```python
from build123d import *

# Parameters (mm, degrees)
EXTRUDE_1_DEPTH          = 70
CUT_EXTRUDE_1_DEPTH      = 100.498743711
SKETCH_4_W               = 45.819685342
SKETCH_4_H               = 5
CUT_EXTRUDE_2_DEPTH      = 96.72878355
SKETCH_5_W               = 32
SKETCH_5_H               = 10
SKETCH_5_H_2             = 40
CUT_EXTRUDE_3_DEPTH      = 94.214805691
CUT_EXTRUDE_4_DEPTH      = 1
SKETCH_7_R               = 3.75
CUT_EXTRUDE_5_DEPTH      = 10
CUT_EXTRUDE_6_REACH      = 97.729
SKETCH_8_R               = 2.5
CUT_EXTRUDE_7_DEPTH      = 92.782351245
CUT_EXTRUDE_7_DEPTH_BACK = 92.782351245
CUT_EXTRUDE_8_DEPTH      = 96
CHAMFER_1_SIZE           = 1


with BuildPart() as part:
    # 草图1 → 拉伸1 (new body)
    with BuildSketch(Plane.XY):
        Polygon((0, 0), (50, 0), (0, 50), align=None)
    extrude(amount=EXTRUDE_1_DEPTH)

    # 草图3 → 切除-拉伸1 (cut, through all)
    with BuildSketch(Plane.XY.offset(70)):
        Polygon((50, 0), (42, 0), (42, 8), align=None)
    extrude(amount=-CUT_EXTRUDE_1_DEPTH, mode=Mode.SUBTRACT)

    # 草图4 → 切除-拉伸2 (cut, through all)
    with BuildSketch(Plane.XY.offset(70)):
        with Locations((32.909842671, 2.5)):
            Rectangle(SKETCH_4_W, SKETCH_4_H)
    extrude(amount=-CUT_EXTRUDE_2_DEPTH, mode=Mode.SUBTRACT)

    # 草图5 → 切除-拉伸3 (cut, through all)
    with BuildSketch(Plane.XZ.offset(-5)):
        with Locations((26, 55)):
            Rectangle(SKETCH_5_W, SKETCH_5_H)
        with Locations((26, 20)):
            Rectangle(SKETCH_5_W, SKETCH_5_H_2)
    extrude(amount=-CUT_EXTRUDE_3_DEPTH, mode=Mode.SUBTRACT)

    # 草图6 → 切除-拉伸4 (cut)
    with BuildSketch(Plane.XY.offset(70)):
        Polygon((0, 50), (0, 30), (20, 30), align=None)
    extrude(amount=-CUT_EXTRUDE_4_DEPTH, mode=Mode.SUBTRACT)

    # 草图7 → 切除-拉伸5 (cut)
    with BuildSketch(Plane.XZ.offset(-5)):
        with Locations(Location((16, 65, 0), (0, 0, 270))):
            Circle(SKETCH_7_R)
    extrude(amount=-CUT_EXTRUDE_5_DEPTH, mode=Mode.SUBTRACT)

    # 切除-拉伸6: up to this face of the body (flat: up to its plane)
    cut_extrude_6_end = Plane(part.part.faces().sort_by_distance((21.50877193, 16.745614035, 40))[0])
    # 草图8 → 切除-拉伸6 (cut, up to the picked face)
    with BuildSketch(Plane.XY.offset(70), mode=Mode.PRIVATE) as cut_extrude_6_sk1:
        with Locations((5, 36)):
            Circle(SKETCH_8_R)
    cut_extrude_6_tool1 = split(extrude(cut_extrude_6_sk1.sketch, amount=-CUT_EXTRUDE_6_REACH, mode=Mode.PRIVATE), bisect_by=cut_extrude_6_end, keep=Keep.BOTH, mode=Mode.PRIVATE)
    # 草图8 → 切除-拉伸6 (cut, up to the picked face)
    with BuildSketch(Plane.XY.offset(70), mode=Mode.PRIVATE) as cut_extrude_6_sk2:
        with Locations((5, 10)):
            Circle(SKETCH_8_R)
    cut_extrude_6_tool2 = split(extrude(cut_extrude_6_sk2.sketch, amount=-CUT_EXTRUDE_6_REACH, mode=Mode.PRIVATE), bisect_by=cut_extrude_6_end, keep=Keep.BOTH, mode=Mode.PRIVATE)
    # 草图8 → 切除-拉伸6 (cut, up to the picked face)
    with BuildSketch(Plane.XY.offset(70), mode=Mode.PRIVATE) as cut_extrude_6_sk3:
        with Locations((31, 10)):
            Circle(SKETCH_8_R)
    cut_extrude_6_tool3 = split(extrude(cut_extrude_6_sk3.sketch, amount=-CUT_EXTRUDE_6_REACH, mode=Mode.PRIVATE), bisect_by=cut_extrude_6_end, keep=Keep.BOTH, mode=Mode.PRIVATE)
    # 草图8 → 切除-拉伸6 (cut, up to the picked face)
    with BuildSketch(Plane.XY.offset(70), mode=Mode.PRIVATE) as cut_extrude_6_sk4:
        with Locations((18, 23)):
            Circle(SKETCH_8_R)
    cut_extrude_6_tool4 = split(extrude(cut_extrude_6_sk4.sketch, amount=-CUT_EXTRUDE_6_REACH, mode=Mode.PRIVATE), bisect_by=cut_extrude_6_end, keep=Keep.BOTH, mode=Mode.PRIVATE)
    add(cut_extrude_6_tool1.solids().sort_by(Axis((5, 36, 70), (0, 0, -1)))[0], mode=Mode.SUBTRACT)
    add(cut_extrude_6_tool2.solids().sort_by(Axis((5, 10, 70), (0, 0, -1)))[0], mode=Mode.SUBTRACT)
    add(cut_extrude_6_tool3.solids().sort_by(Axis((31, 10, 70), (0, 0, -1)))[0], mode=Mode.SUBTRACT)
    add(cut_extrude_6_tool4.solids().sort_by(Axis((18, 23, 70), (0, 0, -1)))[0], mode=Mode.SUBTRACT)

    # 草图9 → 切除-拉伸7 (cut, two sides: drawn at the far end of the back side and taken through both)
    with BuildSketch(Plane(origin=(10, 0, 0), x_dir=(0, 0, -1), z_dir=(1, 0, 0)).offset(-CUT_EXTRUDE_7_DEPTH_BACK)):
        Polygon((182.046505341, 50), (0, 50), (-40, 50), (0, 5), (120.945115134, -131.063254526), (465.924736836, -247.479666759), (527.026127043, -66.416412233), align=None)
    extrude(amount=CUT_EXTRUDE_7_DEPTH + CUT_EXTRUDE_7_DEPTH_BACK, mode=Mode.SUBTRACT)

    # 草图10 → 切除-拉伸8 (cut, through all)
    with BuildSketch(Plane.XY.offset(69)):
        Polygon((0, 50), (0, 47), (3, 47), align=None)
    extrude(amount=-CUT_EXTRUDE_8_DEPTH, mode=Mode.SUBTRACT)

    # 倒角1
    chamfer_1_edges = [part.edges().sort_by_distance(p)[0] for p in [
        (26, 5, 60),
        (26, 5, 50),
        (26, 5, 40),
    ]]
    chamfer(chamfer_1_edges, length=CHAMFER_1_SIZE)


solid = part.part
```
Here's how the part is built. I have some questions about the finished solid (model axes, mm). A direction names the side the tool comes from. Round coordinates to 2 decimals unless told otherwise and drop trailing zeros. Loops run counter-clockwise (first coordinate to the right, second up) from the corner with the lowest first, then second, coordinate; pieces in that order, holes last. Notation, with made-up numbers: (31, 79.25) -> (44, 79.25) arc R24 ccw to (44, 97.25) -> close; hole circle Ø9 at (-7.75, -36). An arc over 180 degrees is marked (long way). Answer as CSV lines item,"result". Start each with the question number.
1. Imagine slicing it at C-C on y = 23. Write out the boundary of the cut face in (x, z), plus the area to 3 significant figures.
2. If we mould it in two halves opening along Y, with no side actions, what happens to faces 4 (the face through (22, 19, 40)), 5 (the face through (4.46, 33.56, 54.7)), 6 (the face through (18, 32, 46)), 7 (the face through (5, 10, 40))? For each: pulls with the +Y half, pulls with the -Y half, needs draft (parallel to the pull), parting line crosses it, or undercut.
3. For faces 1 (the face through (8, 37, 69)), 2 (the face through (5, 36, 40)), 3 (the face through (16, 15, 65)), which set-ups out of +Z, -Z, +X, -X, +Y, -Y let a thin tool reach every point of the face, with its end or its side?
4. I need wall thicknesses on probe 1 along Z at (x, y) = (18.5, 26.5); probe 2 along X at (y, z) = (4, 33); probe 3 along Y at (x, z) = (18, 47). Which ranges of each line are inside material? Lowest first, please. Write a range as from..to.
5. I'm going to push flat-ended pins straight in: P1, Ø20, axis at y = 26.5, z = 44.5, coming from the +X side; P2, Ø4.5, axis at x = 18, y = 23, coming from the +Z side; P3, Ø6, axis at x = 16, z = 65, coming from the -Y side; P4, Ø6, axis at x = 6.5, z = 41, coming from the -Y side. Where does each tip first touch, or does it pass through?
6. Imagine slicing it at B-B on x = 22.5. Write out the boundary of the cut face in (y, z), plus the area to 4 significant figures.
7. Imagine slicing it at A-A on x = 31. Write out the boundary of the cut face in (y, z), plus the area to 4 significant figures.
8. Imagine slicing it at D-D on y = 10. Write out the boundary of the cut face in (x, z), plus the area to 3 significant figures.
Solution:
1,outline,"(0, 16) -> (10, 16) -> (10, 40) -> (15.5, 40) -> (15.5, 50) -> (10, 50) -> (10, 60) -> (15.5, 60) -> (15.5, 70) -> (0, 70) -> close; (20.5, 40) -> (27, 40) -> (27, 50) -> (20.5, 50) -> close; (20.5, 60) -> (27, 60) -> (27, 70) -> (20.5, 70) -> close"
1,area,"780 mm²"
2,face 4,"needs draft"
2,face 5,"undercut"
2,face 6,"pulls with the +Y half"
2,face 7,"undercut"
3,face 1,"+Z, +X, -X, +Y"
3,face 2,"+Z"
3,face 3,"-Y"
4,probe 1,"40..50, 60..70"
4,probe 2,"0..10"
4,probe 3,"5..20.5, 25.5..32"
5,P1,"x = 33.5"
5,P2,"through"
5,P3,"y = 15"
5,P4,"y = 0"
6,outline,"(5, 41) -> (6, 40) -> (27.5, 40) -> (27.5, 50) -> (6, 50) -> (5, 49) -> close; (5, 61) -> (6, 60) -> (27.5, 60) -> (27.5, 70) -> (5, 70) -> close"
6,area,"448.5 mm²"
7,outline,"(5, 41) -> (6, 40) -> (7.5, 40) -> (7.5, 50) -> (6, 50) -> (5, 49) -> close; (5, 61) -> (6, 60) -> (7.5, 60) -> (7.5, 70) -> (5, 70) -> close; (12.5, 40) -> (19, 40) -> (19, 50) -> (12.5, 50) -> close; (12.5, 60) -> (19, 60) -> (19, 70) -> (12.5, 70) -> close"
7,area,"178.5 mm²"
8,outline,"(0, 4.44) -> (10, 4.44) -> (10, 40) -> (28.5, 40) -> (28.5, 50) -> (10, 50) -> (10, 60) -> (28.5, 60) -> (28.5, 70) -> (7.5, 70) -> (7.5, 40) -> (2.5, 40) -> (2.5, 70) -> (0, 70) -> close; (33.5, 40) -> (40, 40) -> (40, 50) -> (33.5, 50) -> close; (33.5, 60) -> (40, 60) -> (40, 70) -> (33.5, 70) -> close; hole circle Ø7.5 at (16, 65)"
8,area,"961 mm²"
